Could you check a few things on this model? Use its own coordinates, in mm. Face numbers are marked on the shaded views. A direction names the side the tool comes from. Round coordinates to 2 decimals unless told otherwise and drop trailing zeros. Loops run counter-clockwise (first coordinate to the right, second up) from the corner with the lowest first, then second, coordinate; pieces in that order, holes last. Notation, with made-up numbers: (8, 27) -> (64, 27) arc R4 ccw to (64, 32) -> close; hole circle Ø4 at (63, 10). An arc over 180 degrees is marked (long way). Put each result on its own line as item: value. Start each with the question number.
1. Imagine slicing it at A-A, the plane z = 2.4. Please give me the cut outline in (x, y) (1 decimal).
2. If we mould it in two halves opening along X, with no side actions, what happens to the marked faces 4 and 5? For each: pulls with the +X half, pulls with the -X half, needs draft (parallel to the pull), parting line crosses it, or undercut.
3. I need wall thicknesses on line 1 (X direction, y = -14, z = 1.15); line 2 (X direction, y = -14.5, z = 4.7); line 3 (X direction, y = 0, z = 3.4). Which ranges of each line are inside material? Lowest first, please. Write a range as [from, to].
4. Which directions (+Z, -Z, +X, -X, +Y, -Y) give clear straight access to the entire face, cutting with the end or side of a thin tool? Please do the marked faces 1, 2 and 3.
5. Imagine slicing it at C-C, the plane x = -27. Please give me the cut outline in (y, z), and give its area (3 significant figures).
6. Imagine slicing it at B-B, the plane y = -27. Please give me the cut outline in (x, z), and give its area (3 significant figures).
7. I'm going to push flat-ended pins straight in: P1, Ø3, axis at y = -5.5, z = 4, coming from the +X side; P2, Ø1.5, axis at x = 19.5, z = 0.5, coming from the +Y side. Where does each tip first touch, or does it pass through?
```python
from build123d import *

# Parameters (mm, degrees)
F1_DEPTH = 5.08
F3_DEPTH = 25.4


# Not quite as in the source:
# - a feature names something its author has since deleted; it is built from what else it names


with BuildPart() as f1:
    # F0 (on Top) → F1 (new body)
    with BuildSketch(Plane.XY):
        with BuildLine():
            Line((6.7351920908, -6.7351920908), (8.9802561211, -8.9802561211))
            ThreePointArc((8.9802561211, -8.9802561211), (10.3222667059, -7.3987032683), (11.3889377966, -5.619795002))
            ThreePointArc((11.3889377966, -5.619795002), (12.3678921005, -2.8853500639), (12.7, 0))
            ThreePointArc((12.7, 0), (-8.9094308211, 9.0505271915), (-0.1995342432, -12.6984324263))
            Line((-0.1995342432, -12.6984324263), (0, -12.1764942784))
            Line((0, -12.1764942784), (0, -4.7625))
            ThreePointArc((0, -4.7625), (-3.3675960454, 3.3675960454), (4.7625, 0))
            ThreePointArc((4.7625, 0), (4.3999762736, -1.8225298466), (3.3675960454, -3.3675960454))
            Line((3.3675960454, -3.3675960454), (4.4901280605, -4.4901280605))
            Line((4.4901280605, -4.4901280605), (6.7351920908, -6.7351920908))
        make_face()
        with BuildLine():
            ThreePointArc((11.3889377966, -5.619795002), (10.3222667059, -7.3987032683), (8.9802561211, -8.9802561211))
            ThreePointArc((8.9802561211, -8.9802561211), (6.8924812287, -10.6669443849), (4.4968663349, -11.8772131902))
            Line((4.4968663349, -11.8772131902), (2.3084511304, -16.9045766677))
            Line((2.3084511304, -16.9045766677), (6.4203654177, -18.6164988404))
            Line((6.4203654177, -18.6164988404), (11.3889377966, -5.619795002))
        make_face()
        with BuildLine():
            Line((2.3084511304, -16.9045766677), (4.4968663349, -11.8772131902))
            ThreePointArc((4.4968663349, -11.8772131902), (2.2857594454, -12.4926099658), (0, -12.7))
            ThreePointArc((0, -12.7), (-0.0997702004, -12.6996081005), (-0.1995342432, -12.6984324263))
            Line((-0.1995342432, -12.6984324263), (-1.2423673122, -15.4262567422))
            Line((-1.2423673122, -15.4262567422), (2.3084511304, -16.9045766677))
        make_face()
        with BuildLine():
            Line((9.2538210972, -19.7961575745), (6.4203654177, -18.6164988404))
            Line((6.4203654177, -18.6164988404), (2.3084511304, -16.9045766677))
            Line((2.3084511304, -16.9045766677), (0.652517293, -20.7086908404))
            Line((0.652517293, -20.7086908404), (10.0662240577, -24.8064846655))
            ThreePointArc((10.0662240577, -24.8064846655), (9.4071650605, -22.3423208774), (9.2538210972, -19.7961575745))
        make_face()
        with BuildLine():
            ThreePointArc((-0.1995342432, -12.6984324263), (-0.0997702004, -12.6996081005), (0, -12.7))
            Line((0, -12.7), (0, -12.1764942784))
            Line((0, -12.1764942784), (-0.1995342432, -12.6984324263))
        make_face()
        with BuildLine():
            Line((0.652517293, -20.7086908404), (2.3084511304, -16.9045766677))
            Line((2.3084511304, -16.9045766677), (-1.2423673122, -15.4262567422))
            Line((-1.2423673122, -15.4262567422), (-15.757129186, -9.3832945241))
            ThreePointArc((-15.757129186, -9.3832945241), (-13.5731230118, -10.5544783892), (-11.6581465409, -12.1275072291))
            ThreePointArc((-11.6581465409, -12.1275072291), (-9.971458277, -14.2152821214), (-8.7611894717, -16.6108970152))
            Line((-8.7611894717, -16.6108970152), (0.652517293, -20.7086908404))
        make_face()
        with BuildLine():
            Line((18.5758412025, -23.677214376), (9.2538210972, -19.7961575745))
            ThreePointArc((9.2538210972, -19.7961575745), (9.4071650605, -22.3423208774), (10.0662240577, -24.8064846655))
            Line((10.0662240577, -24.8064846655), (15.2082451571, -27.0448104214))
            Line((15.2082451571, -27.0448104214), (17.4533091874, -24.7997463911))
            Line((17.4533091874, -24.7997463911), (18.5758412025, -23.677214376))
        make_face()
        with BuildLine():
            ThreePointArc((34.6434372479, -20.3096183306), (22.2002201194, -7.6122145583), (9.2538210972, -19.7961575745))
            Line((9.2538210972, -19.7961575745), (18.5758412025, -23.677214376))
            ThreePointArc((18.5758412025, -23.677214376), (20.1209074013, -15.909642057), (26.7059372479, -20.3096183306))
            ThreePointArc((26.7059372479, -20.3096183306), (25.3110332933, -23.677214376), (21.9434372479, -25.0721183306))
            Line((21.9434372479, -25.0721183306), (21.9434372479, -33.0096183306))
            ThreePointArc((21.9434372479, -33.0096183306), (30.923693369, -29.2898744517), (34.6434372479, -20.3096183306))
        make_face()
        with BuildLine():
            Line((10.0662240577, -24.8064846655), (0.652517293, -20.7086908404))
            Line((0.652517293, -20.7086908404), (-8.7611894717, -16.6108970152))
            ThreePointArc((-8.7611894717, -16.6108970152), (-8.1457926961, -18.8220039048), (-7.9384026619, -21.1077633501))
            ThreePointArc((-7.9384026619, -21.1077633501), (-7.9409988896, -21.3645462216), (-7.9487865112, -21.6212241063))
            Line((-7.9487865112, -21.6212241063), (17.062163772, -32.0340871567))
            ThreePointArc((17.062163772, -32.0340871567), (14.8781575978, -30.8629032915), (12.9631811269, -29.2898744517))
            ThreePointArc((12.9631811269, -29.2898744517), (11.276492863, -27.2020995593), (10.0662240577, -24.8064846655))
        make_face()
        with BuildLine():
            ThreePointArc((21.9434372479, -25.0721183306), (20.1209074013, -24.7095946042), (18.5758412025, -23.677214376))
            Line((18.5758412025, -23.677214376), (17.4533091874, -24.7997463911))
            Line((17.4533091874, -24.7997463911), (15.2082451571, -27.0448104214))
            Line((15.2082451571, -27.0448104214), (12.9631811269, -29.2898744517))
            ThreePointArc((12.9631811269, -29.2898744517), (14.8781575978, -30.8629032915), (17.062163772, -32.0340871567))
            ThreePointArc((17.062163772, -32.0340871567), (19.4545372993, -32.7633477739), (21.9434372479, -33.0096183306))
            Line((21.9434372479, -33.0096183306), (21.9434372479, -25.0721183306))
        make_face()
        with BuildLine():
            ThreePointArc((-11.6581465409, -12.1275072291), (-13.5731230118, -10.5544783892), (-15.757129186, -9.3832945241))
            ThreePointArc((-15.757129186, -9.3832945241), (-31.3447452065, -27.9388854628), (-7.9487865112, -21.6212241063))
            Line((-7.9487865112, -21.6212241063), (-9.1820824244, -21.1077633501))
            Line((-9.1820824244, -21.1077633501), (-15.8759026619, -21.1077633501))
            ThreePointArc((-15.8759026619, -21.1077633501), (-25.0383789355, -22.9302931968), (-17.2708066165, -17.7401673047))
            Line((-17.2708066165, -17.7401673047), (-16.1482746014, -16.6176352896))
            Line((-16.1482746014, -16.6176352896), (-13.9032105711, -14.3725712593))
            Line((-13.9032105711, -14.3725712593), (-11.6581465409, -12.1275072291))
        make_face()
        with BuildLine():
            Line((-9.1820824244, -21.1077633501), (-7.9487865112, -21.6212241063))
            ThreePointArc((-7.9487865112, -21.6212241063), (-7.9409988896, -21.3645462216), (-7.9384026619, -21.1077633501))
            Line((-7.9384026619, -21.1077633501), (-9.1820824244, -21.1077633501))
        make_face()
        with BuildLine():
            Line((15.2082451571, -27.0448104214), (10.0662240577, -24.8064846655))
            ThreePointArc((10.0662240577, -24.8064846655), (11.276492863, -27.2020995593), (12.9631811269, -29.2898744517))
            Line((12.9631811269, -29.2898744517), (15.2082451571, -27.0448104214))
        make_face()
        with BuildLine():
            ThreePointArc((0, -12.7), (2.2857594454, -12.4926099658), (4.4968663349, -11.8772131902))
            Line((4.4968663349, -11.8772131902), (6.7351920908, -6.7351920908))
            Line((6.7351920908, -6.7351920908), (4.4901280605, -4.4901280605))
            Line((4.4901280605, -4.4901280605), (3.3675960454, -3.3675960454))
            Line((3.3675960454, -3.3675960454), (0, -12.1764942784))
            Line((0, -12.1764942784), (0, -12.7))
        make_face()
        with BuildLine():
            Line((-15.8759026619, -21.1077633501), (-9.1820824244, -21.1077633501))
            Line((-9.1820824244, -21.1077633501), (-17.2708066165, -17.7401673047))
            ThreePointArc((-17.2708066165, -17.7401673047), (-16.2384263884, -19.2852335035), (-15.8759026619, -21.1077633501))
        make_face()
        with BuildLine():
            ThreePointArc((-7.9384026619, -21.1077633501), (-8.1457926961, -18.8220039048), (-8.7611894717, -16.6108970152))
            Line((-8.7611894717, -16.6108970152), (-13.9032105711, -14.3725712593))
            Line((-13.9032105711, -14.3725712593), (-16.1482746014, -16.6176352896))
            Line((-16.1482746014, -16.6176352896), (-17.2708066165, -17.7401673047))
            Line((-17.2708066165, -17.7401673047), (-9.1820824244, -21.1077633501))
            Line((-9.1820824244, -21.1077633501), (-7.9384026619, -21.1077633501))
        make_face()
        with BuildLine():
            Line((0, -4.7625), (0, -12.1764942784))
            Line((0, -12.1764942784), (3.3675960454, -3.3675960454))
            ThreePointArc((3.3675960454, -3.3675960454), (1.8225298466, -4.3999762736), (0, -4.7625))
        make_face()
        with BuildLine():
            Line((-13.9032105711, -14.3725712593), (-8.7611894717, -16.6108970152))
            ThreePointArc((-8.7611894717, -16.6108970152), (-9.971458277, -14.2152821214), (-11.6581465409, -12.1275072291))
            Line((-11.6581465409, -12.1275072291), (-13.9032105711, -14.3725712593))
        make_face()
        with BuildLine():
            ThreePointArc((4.4968663349, -11.8772131902), (6.8924812287, -10.6669443849), (8.9802561211, -8.9802561211))
            Line((8.9802561211, -8.9802561211), (6.7351920908, -6.7351920908))
            Line((6.7351920908, -6.7351920908), (4.4968663349, -11.8772131902))
        make_face()
    extrude(amount=F1_DEPTH)

    # F2 (on face) → F3 (cut)
    with BuildSketch(Plane.XY.offset(5.08)):
        with BuildLine():
            Line((-15.8846679825, -20.8189505253), (-8.3298662663, -24.2366500209))
            ThreePointArc((-8.3298662663, -24.2366500209), (-8.0711029973, -22.9388775299), (-7.9487865112, -21.6212241063))
            Line((-7.9487865112, -21.6212241063), (-18.6754288181, -16.7686228893))
            ThreePointArc((-18.6754288181, -16.7686228893), (-16.7166897918, -18.4056207903), (-15.8846679825, -20.8189505253))
        make_face()
        with BuildLine():
            ThreePointArc((-2.823583262, -12.3821394582), (-1.5198092555, -12.6087342674), (-0.1995342432, -12.6984324263))
            Line((-0.1995342432, -12.6984324263), (4.3863512165, -1.8550820077))
            ThreePointArc((4.3863512165, -1.8550820077), (2.7982865403, -3.8536993511), (0.406267641, -4.7451399193))
            Line((0.406267641, -4.7451399193), (-2.823583262, -12.3821394582))
        make_face()
        with BuildLine():
            ThreePointArc((9.6349008523, -17.1807316599), (9.3761375833, -18.4785041508), (9.2538210972, -19.7961575745))
            Line((9.2538210972, -19.7961575745), (19.9804634041, -24.6487587914))
            ThreePointArc((19.9804634041, -24.6487587914), (18.0217243778, -23.0117608905), (17.1897025685, -20.5984311555))
            Line((17.1897025685, -20.5984311555), (9.6349008523, -17.1807316599))
        make_face()
    extrude(amount=-F3_DEPTH, mode=Mode.SUBTRACT)


solid = f1.part
```
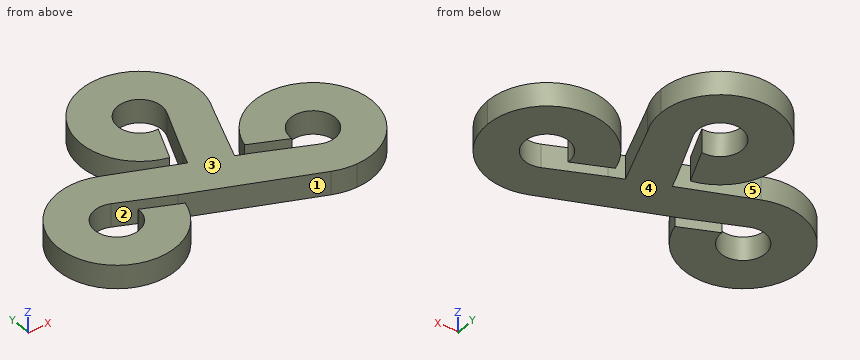
Entries:
1. outline: (-18.7, -16.8) -> (-7.9, -21.6) -> (17.1, -32) arc R12.7 ccw (long way) to (9.6, -17.2) -> (17.2, -20.6) arc R4.8 cw (long way) to (20, -24.6) -> (9.3, -19.8) -> (6.4, -18.6) -> (11.4, -5.6) arc R12.7 ccw (long way) to (-2.8, -12.4) -> (0.4, -4.7) arc R4.8 cw (long way) to (4.4, -1.9) -> (-0.2, -12.7) -> (-1.2, -15.4) -> (-15.8, -9.4) arc R12.7 ccw (long way) to (-8.3, -24.2) -> (-15.9, -20.8) arc R4.8 cw (long way) to start
2. face 4: needs draft
2. face 5: undercut
3. line 1: [-31.16, -4.67], [-0.7, 8.19], [10.92, 32.97]
3. line 2: [-31.48, -3.47], [-0.89, 7.99], [10.65, 33.24]
3. line 3: [-12.7, -4.76], [4.76, 12.7]
4. face 1: +Z, -Z, -Y
4. face 2: +Z, -Z
4. face 3: +Z, +X, -X, +Y, -Y
5. outline: (-32.1, 0) -> (-10.12, 0) -> (-10.12, 5.08) -> (-32.1, 5.08) -> close
5. area: 112 mm^2
6. outline: (-31.89, 0) -> (-9.39, 0) -> (-9.39, 5.08) -> (-31.89, 5.08) -> close; (4.97, 0) -> (32.74, 0) -> (32.74, 5.08) -> (4.97, 5.08) -> close
6. area: 255 mm^2
7. P1: x = 12.05
7. P2: y = -7.72
